```python
from build123d import *

# Parameters (mm, degrees)
SKETCH_W        = 244
SKETCH_H        = 70
PAD_DEPTH       = 10
FILLET_R        = 3
FILLET001_R     = 3
FILLET002_R     = 3
FILLET003_R     = 3
POCKET_DEPTH    = 5
SKETCH002_W     = 10
SKETCH002_H     = 10
POCKET001_DEPTH = 10.001
SKETCH003_R     = 3.5
SKETCH003_R_2   = 3.25
SKETCH003_R_3   = 2
POCKET002_DEPTH = 10.001
SKETCH004_W     = 45
SKETCH004_H     = 12
POCKET003_DEPTH = 5
FILLET004_R     = 2
FILLET005_R     = 2
FILLET006_R     = 2
FILLET007_R     = 2


with BuildPart() as part:
    # Sketch → Pad (new body)
    with BuildSketch(Plane.XY):
        Rectangle(SKETCH_W, SKETCH_H)
    extrude(amount=PAD_DEPTH)

    # Fillet
    fillet_edges = [part.edges().sort_by_distance(p)[0] for p in [
        (0, -35, 10),
    ]]
    fillet(fillet_edges, radius=FILLET_R)

    # Fillet001
    fillet001_edges = [part.edges().sort_by_distance(p)[0] for p in [
        (-122, 1.5, 10),
    ]]
    fillet(fillet001_edges, radius=FILLET001_R)

    # Fillet002
    fillet002_edges = [part.edges().sort_by_distance(p)[0] for p in [
        (1.5, 35, 10),
    ]]
    fillet(fillet002_edges, radius=FILLET002_R)

    # Fillet003
    fillet003_edges = [part.edges().sort_by_distance(p)[0] for p in [
        (122, 0, 10),
    ]]
    fillet(fillet003_edges, radius=FILLET003_R)

    # Sketch001 (on Face2 of Fillet003) → Pocket (cut)
    with BuildSketch(Plane(origin=(0, 0, 0), x_dir=(1, 0, 0), z_dir=(0, 0, -1))):
        with BuildLine():
            ThreePointArc((-117, 30), (-119.5, 27.5), (-117, 25))
            Line((-117, 25), (117, 25))
            ThreePointArc((117, 25), (119.5, 27.5), (117, 30))
            Line((-117, 30), (117, 30))
        make_face()
        with BuildLine():
            ThreePointArc((-117, -25), (-119.5, -27.5), (-117, -30))
            Line((-117, -30), (117, -30))
            ThreePointArc((117, -30), (119.5, -27.5), (117, -25))
            Line((-117, -25), (117, -25))
        make_face()
    extrude(amount=-POCKET_DEPTH, mode=Mode.SUBTRACT)

    # Sketch002 (on Face2 of Pocket) → Pocket001 (cut, through all)
    with BuildSketch(Plane(origin=(0, 0, 0), x_dir=(1, 0, 0), z_dir=(0, 0, -1))):
        with Locations((-117, 10)):
            Rectangle(SKETCH002_W, SKETCH002_H)
        with Locations((-117, 30)):
            Rectangle(SKETCH002_W, SKETCH002_H)
        with Locations((-117, -10)):
            Rectangle(SKETCH002_W, SKETCH002_H)
        with Locations((117, 10)):
            Rectangle(SKETCH002_W, SKETCH002_H)
        with Locations((117, 30)):
            Rectangle(SKETCH002_W, SKETCH002_H)
        with Locations((117, -10)):
            Rectangle(SKETCH002_W, SKETCH002_H)
        with Locations((-117, -30)):
            Rectangle(SKETCH002_W, SKETCH002_H)
        with Locations((117, -30)):
            Rectangle(SKETCH002_W, SKETCH002_H)
    extrude(amount=-POCKET001_DEPTH, mode=Mode.SUBTRACT)

    # Sketch003 (on Face2 of Pocket001) → Pocket002 (cut, through all)
    with BuildSketch(Plane(origin=(0, 0, 0), x_dir=(1, 0, 0), z_dir=(0, 0, -1))):
        with Locations((90, 0)):
            Circle(SKETCH003_R)
        with Locations((65, 0)):
            Circle(SKETCH003_R_2)
        with Locations((-85, 0)):
            Circle(SKETCH003_R_3)
        with Locations((35, 0)):
            Circle(SKETCH003_R_3)
    extrude(amount=-POCKET002_DEPTH, mode=Mode.SUBTRACT)

    # Sketch004 (on Face2 of Pocket002) → Pocket003 (cut)
    with BuildSketch(Plane(origin=(0, 0, 0), x_dir=(1, 0, 0), z_dir=(0, 0, -1))):
        with Locations((77.5, 0)):
            Rectangle(SKETCH004_W, SKETCH004_H)
    extrude(amount=-POCKET003_DEPTH, mode=Mode.SUBTRACT)

    # Fillet004
    fillet004_edges = [part.edges().sort_by_distance(p)[0] for p in [
        (100, 6, 2.5),
    ]]
    fillet(fillet004_edges, radius=FILLET004_R)

    # Fillet005
    fillet005_edges = [part.edges().sort_by_distance(p)[0] for p in [
        (55, 6, 2.5),
    ]]
    fillet(fillet005_edges, radius=FILLET005_R)

    # Fillet006
    fillet006_edges = [part.edges().sort_by_distance(p)[0] for p in [
        (55, -6, 2.5),
    ]]
    fillet(fillet006_edges, radius=FILLET006_R)

    # Fillet007
    fillet007_edges = [part.edges().sort_by_distance(p)[0] for p in [
        (100, -6, 2.5),
    ]]
    fillet(fillet007_edges, radius=FILLET007_R)


with BuildPart() as part_1:
    # Body placement: moved
    add(part.part.moved(Location((140, -80, 0))))


solid = part_1.part
```
Input: part model. Units: mm. Frame: model coordinates. A direction names the side the tool comes from. Coordinates: 2 decimals unless noted, no trailing zeros. Write each loop counter-clockwise with the first axis right and the second up, starting at its lowest first coordinate (ties: lowest second). Pieces come first, ordered by that corner, then holes. Notation, with made-up numbers: M 82.25,72.5 L 140.25,72.5 A23 cw 140.25,99.5 Z; hole C -34,-25.5 d6. An arc over 180 degrees is marked long. Use one line per item in the form item = value.
Q1. Draft query along X for faces 1 (the face through (138, -112, 0)), 2 (the face through (262, -60, 3)), 3 (the face through (195, -80, 2)), 4 (the face through (173.526, -81.352, 4.93)). Return one class per face: released by +X, released by -X, zero draft, split by the parting line, or undercut.
Answer below:
face_1 = zero draft
face_2 = released by +X
face_3 = undercut
face_4 = undercut
Q2. Section C-C (z = 2). Count the separate pieces of the cut face and the enclosed holes in it, plus the area to 3 significant figures.
Answer below:
separate_pieces = 3
enclosed_holes = 3
area = 13,500 mm²
Q3. Section A-A (x = 205). Return loops of the section in (y, z), plus the area to 3 significant figures.
Answer below:
outline = M -115,0 L -110,0 L -110,5 L -105,5 L -105,0 L -86,0 L -86,5 L -83.25,5 L -83.25,10 L -112,10 A3 ccw -115,7 Z; M -76.75,5 L -74,5 L -74,0 L -55,0 L -55,5 L -50,5 L -50,0 L -45,0 L -45,7 A3 ccw -48,10 L -76.75,10 Z
area = 554 mm²
Q4. Set-up query: faces 5 (the face through (23, -75, 5)), 6 (the face through (252, -49, 6)), 7 (the face through (28, -111, 6)). Return all of +Z, -Z, +X, -X, +Y, -Y with unobstructed straight access to the full face (end or side cutting, diameter ignored); none if empty.
Answer below:
face_5 = +Z, -Z, -X
face_6 = +Z, -Z, +X, +Y
face_7 = +Z, -Z, -X, -Y
Q5. First-contact query: pin 1 (1.5 mm diameter, centred on x = 113.5, z = 9, fed in from +Y); pin 2 (3 mm diameter, centred on x = 258, z = 4, fed in from +Y); pin 3 (5.5 mm diameter, centred on x = 157, y = -52, fed in from -Z); pin 4 (3 mm diameter, centred on y = -71, z = 3, fed in from -X). Flat tips, straight axial feed; report the tip coordinate or a pass-through.
Answer below:
pin_1 = -45.27
pin_2 = -55
pin_3 = 0
pin_4 = 28
Q6. Section B-B (x = 40.5). Return loops of the section in (y, z), plus the area to 3 significant figures.
Answer below:
outline = M -115,0 L -110,0 L -110,5 L -105,5 L -105,0 L -55,0 L -55,5 L -50,5 L -50,0 L -45,0 L -45,7 A3 ccw -48,10 L -112,10 A3 ccw -115,7 Z
area = 646 mm²
Q7. Material intervals for probe 1 along X at (y, z) = (-80, 4.5); probe 2 along Y at (x, z) = (119, 3.25); probe 3 along Y at (x, z) = (55, 4), sorted ascending. Write a range as from..to.
Answer below:
probe_1 = 18..53, 57..173, 177..195, 240..262
probe_2 = -115..-110, -105..-55, -50..-45
probe_3 = -115..-110, -105..-82, -78..-55, -50..-45
Q8. Section D-D (x = 230). Return loops of the section in (y, z).
Answer below:
outline = M -115,0 L -110,0 L -110,5 L -105,5 L -105,0 L -86,0 L -86,5 L -83.5,5 L -83.5,10 L -112,10 A3 ccw -115,7 Z; M -76.5,5 L -74,5 L -74,0 L -55,0 L -55,5 L -50,5 L -50,0 L -45,0 L -45,7 A3 ccw -48,10 L -76.5,10 Z
